Here's how the part is built. I have some questions about the finished solid (model axes, mm). Face numbers are marked on the shaded views. A direction names the side the tool comes from. Coordinates: 2 decimals unless noted, no trailing zeros. Loops run counter-clockwise (first coordinate to the right, second up) from the corner with the lowest first, then second, coordinate; pieces in that order, holes last. Notation, with made-up numbers: (56.5, 71) -> (74.5, 71) arc R26 ccw to (74.5, 100) -> close; hole circle Ø4 at (60.5, -16). An arc over 180 degrees is marked (long way). Answer as a JSON object with one key per item and string values. Group by question number.
1) I want a section at C-C (y = -1.25). Write out the boundary of the cut face in (x, z), then the cut area to 4 significant figures.
2) I need wall thicknesses on probe 1 along X at (y, z) = (1.75, 17); probe 2 along Y at (x, z) = (3, -11); probe 3 along Z at (x, y) = (5, -2.75). Which ranges of each line are inside material? Lowest first, please. Write a range as [from, to].
3) If we mould it in two halves opening along Z, with no side actions, what happens to the marked faces 1, 2 and 3? For each: +Z half, -Z half, draft (parallel to the pull), parting line (faces both ways), or undercut.
4) I'm going to push flat-ended pins straight in: pin 1 (2.5 mm diameter, centred on y = 5.5, z = 4, fed in from +X); pin 2 (1 mm diameter, centred on x = 10, z = 6.5, fed in from +Y); pin 3 (2 mm diameter, centred on x = -26, z = 17, fed in from +Y); pin 4 (6 mm diameter, centred on y = 10.5, z = 24, fed in from +X). Where does each tip first touch, or does it pass through?
5) Which directions (+Z, -Z, +X, -X, +Y, -Y) give clear straight access to the entire face, cutting with the end or side of a thin tool? Please do the marked faces 4, 5, 6 and 7.
6) I want a section at A-A (y = 5.25). Count the separate pieces of the cut face and the enclosed holes in it, then the cut area to 3 significant figures.
7) I want a section at B-B (x = 16.5). Write out the boundary of the cut face in (y, z).
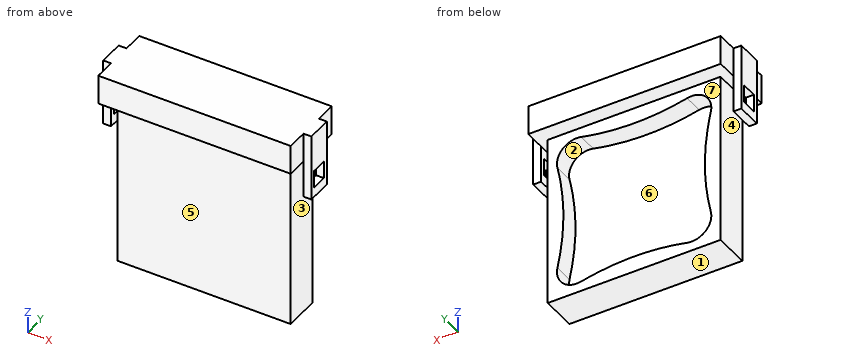
```python
from build123d import *

# Parameters (mm, degrees)
SKETCH1_W           = 44
SKETCH1_H           = 44
BOSS_EXTRUDE1_DEPTH = 9
SKETCH2_W           = 49
SKETCH2_H           = 17
BOSS_EXTRUDE2_DEPTH = 7.5
CUT_EXTRUDE1_DEPTH  = 5
SKETCH4_W           = 4.5
SKETCH4_H           = 4
BOSS_EXTRUDE3_DEPTH = 2


with BuildPart() as part:
    # Sketch1 → Boss-Extrude1 (new body)
    with BuildSketch(Plane(origin=(0, 0, 0), x_dir=(1, 0, 0), z_dir=(0, 1, 0))):
        Rectangle(SKETCH1_W, SKETCH1_H)
    extrude(amount=BOSS_EXTRUDE1_DEPTH)

    # Sketch2 → Boss-Extrude2 (add)
    with BuildSketch(Plane.XY.offset(22)):
        with Locations((0, 4.5)):
            Rectangle(SKETCH2_W, SKETCH2_H)
    extrude(amount=BOSS_EXTRUDE2_DEPTH)

    # Sketch3 → Cut-Extrude1 (cut)
    with BuildSketch(Plane(origin=(0, 9, 0), x_dir=(1, 0, 0), z_dir=(0, 1, 0))):
        with BuildLine():
            ThreePointArc((-19.5325, -13.495), (-18.170661955, -18.166166123), (-13.49, -19.495))
            add(Edge.make_bspline(
                [(-13.49, -19.495), (-4.496666667, -17.441666667), (4.496666667, -17.441666667), (13.49, -19.495)],
                knots=[0, 0, 0, 0, 1, 1, 1, 1], degree=3))
            ThreePointArc((13.49, -19.495), (18.162524477, -18.157971004), (19.5325, -13.495))
            add(Edge.make_bspline(
                [(19.5325, 13.495), (16.4925, 0), (19.5325, -13.495)],
                knots=[0, 0, 0, 1, 1, 1], degree=2))
            ThreePointArc((19.5325, 13.495), (18.162524477, 18.157971004), (13.49, 19.495))
            add(Edge.make_bspline(
                [(-13.49, 19.495), (-4.496666667, 17.441666667), (4.496666667, 17.441666667), (13.49, 19.495)],
                knots=[0, 0, 0, 0, 1, 1, 1, 1], degree=3))
            ThreePointArc((-13.49, 19.495), (-18.170661955, 18.166166123), (-19.5325, 13.495))
            add(Edge.make_bspline(
                [(-19.5325, 13.495), (-18.519166667, 8.996666667), (-17.505833333, 0), (-18.519166667, -8.996666667), (-19.5325, -13.495)],
                knots=[0, 0, 0, 0, 0.5, 1, 1, 1, 1], degree=3))
        make_face()
    extrude(amount=-CUT_EXTRUDE1_DEPTH, mode=Mode.SUBTRACT)

    # Sketch4 → Boss-Extrude3 (add)
    with BuildSketch(Plane(origin=(24.5, 0, 0), x_dir=(0, 0, -1), z_dir=(1, 0, 0))):
        Polygon((-29.5, 4.5), (-29.5, 7.7), (-12.5, 7.7), (-12.5, 1.3), (-29.5, 1.3), align=None)
        with Locations((-17.25, 4.5)):
            Rectangle(SKETCH4_W, SKETCH4_H, mode=Mode.SUBTRACT)
    boss_extrude3 = extrude(amount=BOSS_EXTRUDE3_DEPTH)

    # Mirror1: Boss-Extrude3 across plane
    add(boss_extrude3.mirror(Plane(origin=(0, 0, 0), x_dir=(0, 0, 1), z_dir=(1, 0, 0))))


solid = part.part
```
Determined:
{
 "1": {"outline": "(-24.5, 22) -> (24.5, 22) -> (24.5, 29.5) -> (-24.5, 29.5) -> close", "area": "367.5 mm^2"},
 "2": {"probe 1": "[-26.5, -24.5], [-22, 22], [24.5, 26.5]", "probe 2": "[0, 4]", "probe 3": "[22, 29.5]"},
 "3": {"face 1": "-Z half", "face 2": "undercut", "face 3": "draft"},
 "4": {"pin 1": "x = 22", "pin 2": "y = 4", "pin 3": "y = 7.7", "pin 4": "x = 26.5"},
 "5": {"face 4": "-Z, +Y, -Y", "face 5": "-Z, +X, -X, -Y", "face 6": "+Y", "face 7": "-Z, +X, -X, +Y"},
 "6": {"separate pieces": "3", "enclosed holes": "1", "area": "956 mm^2"},
 "7": {"outline": "(-4, 22) -> (0, 22) -> (0, -22) -> (9, -22) -> (9, -19.25) -> (4, -19.25) -> (4, 19.25) -> (9, 19.25) -> (9, 22) -> (13, 22) -> (13, 29.5) -> (-4, 29.5) -> close"}
}
